```python
from build123d import *
from build123d.topology import SkipClean

# Parameters (mm, degrees)
SKETCH_1_R          = 1.55
SKETCH_1_R_2        = 4
EXTRUDE_1_DEPTH     = 3
EXTRUDE_START       = -3
SKETCH_2_R          = 2.1
EXTRUDE_3_DEPTH     = 3
FILLET_1_R          = 4
FILLET_2_R          = 314
FILLET_3_R          = 314
FILLET_4_R          = 4
CUT_EXTRUDE_2_DEPTH = 3
EXTRUDE_4_DEPTH     = 3
EXTRUDE_5_DEPTH     = 3
SKETCH_6_R          = 1.55
CUT_EXTRUDE_3_DEPTH = 10


with BuildPart() as part:
    # 草图1 → 凸台-拉伸1 (new body)
    with BuildSketch(Plane(origin=(0, 0, 0), x_dir=(1, 0, 0), z_dir=(0, 1, 0))):
        with BuildLine():
            Line((-27.819418646, 37.14796354), (-55, 11))
            Line((-55, 11), (-55, -11))
            Line((-55, -11), (-27.819418646, -37.14796354))
            ThreePointArc((-27.819418646, -37.14796354), (-23.984664844, -39.630488814), (-19.5, -40.5))
            Line((-19.5, -40.5), (-17.421399483, -40.31860482))
            Line((-17.421399483, -40.31860482), (45.042813224, -34.867481809))
            ThreePointArc((45.042813224, -34.867481809), (58.724014778, -30.74585061), (69.617928959, -21.5))
            Line((69.617928959, -21.5), (19, -21.5))
            ThreePointArc((19, -21.5), (15.464466094, -20.035533906), (14, -16.5))
            Line((14, -16.5), (14, -12.539936204))
            ThreePointArc((14, -12.539936204), (5.5, 0), (14, 12.539936204))
            Line((14, 12.539936204), (14, 16.5))
            ThreePointArc((14, 16.5), (15.464466094, 20.035533906), (19, 21.5))
            Line((19, 21.5), (69.617928959, 21.5))
            ThreePointArc((69.617928959, 21.5), (58.724014778, 30.74585061), (45.042813224, 34.867481809))
            Line((45.042813224, 34.867481809), (-17.421399483, 40.31860482))
            Line((-17.421399483, 40.31860482), (-19.5, 40.5))
            ThreePointArc((-19.5, 40.5), (-23.984664844, 39.630488814), (-27.819418646, 37.14796354))
        make_face()
        with Locations(Location((-29, -28.5, 0), (0, 0, 270))):
            Circle(SKETCH_1_R, mode=Mode.SUBTRACT)
        with Locations(Location((-19.5, -36.5, 0), (0, 0, 270))):
            Circle(SKETCH_1_R, mode=Mode.SUBTRACT)
        with Locations(Location((-19.5, -28.5, 0), (0, 0, 270))):
            Circle(SKETCH_1_R_2, mode=Mode.SUBTRACT)
        with Locations(Location((-10, -28.5, 0), (0, 0, 270))):
            Circle(SKETCH_1_R, mode=Mode.SUBTRACT)
        with Locations(Location((-19.5, -20.5, 0), (0, 0, 270))):
            Circle(SKETCH_1_R, mode=Mode.SUBTRACT)
        with Locations(Location((-46.5, 0, 0), (0, 0, 270))):
            Circle(SKETCH_1_R, mode=Mode.SUBTRACT)
        with Locations(Location((-27.5, 0, 0), (0, 0, 270))):
            Circle(SKETCH_1_R, mode=Mode.SUBTRACT)
        with Locations(Location((0, 0, 0), (0, 0, 270))):
            Circle(SKETCH_1_R, mode=Mode.SUBTRACT)
        with Locations(Location((-29, 28.5, 0), (0, 0, 270))):
            Circle(SKETCH_1_R, mode=Mode.SUBTRACT)
        with Locations(Location((-19.5, 20.5, 0), (0, 0, 270))):
            Circle(SKETCH_1_R, mode=Mode.SUBTRACT)
        with Locations(Location((-19.5, 28.5, 0), (0, 0, 270))):
            Circle(SKETCH_1_R_2, mode=Mode.SUBTRACT)
        with Locations(Location((-10, 28.5, 0), (0, 0, 270))):
            Circle(SKETCH_1_R, mode=Mode.SUBTRACT)
        with Locations(Location((-19.5, 36.5, 0), (0, 0, 270))):
            Circle(SKETCH_1_R, mode=Mode.SUBTRACT)
    extrude(amount=EXTRUDE_1_DEPTH)

    # 草图2 → 凸台-拉伸3 (add)
    with BuildSketch(Plane(origin=(0, 3, 0), x_dir=(1, 0, 0), z_dir=(0, 1, 0)).offset(EXTRUDE_START)):
        with BuildLine():
            Line((-7, 60), (-28.363974347, 36.588878709))
            ThreePointArc((-28.363974347, 36.588878709), (-26.665503977, 38.125775437), (-24.705947863, 39.311942788))
            Line((-24.705947863, 39.311942788), (-19.656872495, 39.177623495))
            Line((-19.656872495, 39.177623495), (-17.421399483, 40.31860482))
            Line((-17.421399483, 40.31860482), (17, 37.314720281))
            Line((17, 37.314720281), (17, 50))
            Line((17, 50), (17, 60))
            Line((17, 60), (-7, 60))
        make_face()
        with Locations(Location((13, 55, 0), (0, 0, 270))):
            Circle(SKETCH_2_R, mode=Mode.SUBTRACT)
        with Locations(Location((-3, 55, 0), (0, 0, 270))):
            Circle(SKETCH_2_R, mode=Mode.SUBTRACT)
    extrude_3 = extrude(amount=EXTRUDE_3_DEPTH)

    # 圆角1
    fillet_1_edges = [part.edges().sort_by_distance(p)[0] for p in [
        (17, 1.5, -37.314720281),
    ]]
    fillet(fillet_1_edges, radius=FILLET_1_R)

    # 圆角2
    # the kernel refuses this fillet: 314 mm, written as the material it adds along each edge
    with BuildSketch(Plane(origin=(-28.100791786, 0, -36.877280051), x_dir=(0.6740732257670936, 0, -0.7386645289330906), z_dir=(0, 1, 0))) as fillet_2_piece_1:
        with BuildLine():
            CenterArc((FILLET_2_R * 0.032536346624, FILLET_2_R), FILLET_2_R, 266.272924122, 3.727075878)
            Line((-FILLET_2_R * 0.0324675326171, FILLET_2_R * 0.0021149887469), (0, 0))
            Line((0, 0), (FILLET_2_R * 0.032536346624, 0))
        make_face()
    extrude(amount=3)

    # 镜向2: 凸台-拉伸3 across plane
    add(extrude_3.mirror(Plane.XY))

    # 圆角3
    # the kernel refuses this fillet: 314 mm, written as the material it adds along each edge
    with BuildSketch(Plane(origin=(-28.100791786, 0, 36.877280051), x_dir=(-0.7206636283184775, 0, -0.6932848871992288), z_dir=(0, 1, 0))) as fillet_3_piece_1:
        with BuildLine():
            CenterArc((FILLET_3_R * 0.0325363466241, FILLET_3_R), FILLET_3_R, 266.272924122, 3.727075878)
            Line((-FILLET_3_R * 0.0324675326171, FILLET_3_R * 0.0021149887469), (0, 0))
            Line((0, 0), (FILLET_3_R * 0.032536346624, 0))
        make_face()
    extrude(amount=3)

    # 圆角4
    fillet_4_edges = [part.edges().sort_by_distance(p)[0] for p in [
        (17, 1.5, 37.314720281),
    ]]
    fillet(fillet_4_edges, radius=FILLET_4_R)

    # 草图3 → 切除-拉伸2 (cut)
    with BuildSketch(Plane.XZ):
        with BuildLine():
            ThreePointArc((-8.686732059, 48.231275591), (-35.637539634, 44.178960889), (-38.911435654, 17.122558906))
            ThreePointArc((-38.911435654, 17.122558906), (-32.411561674, 15.426493388), (-30.715496156, 21.926367368))
            ThreePointArc((-30.715496156, 21.926367368), (-28.823911789, 37.55895518), (-13.252334078, 39.900292563))
            ThreePointArc((-13.252334078, 39.900292563), (-6.804041555, 41.782983067), (-8.686732059, 48.231275591))
        make_face()
    cut_extrude_2 = extrude(amount=-CUT_EXTRUDE_2_DEPTH, mode=Mode.SUBTRACT)

    # 草图4 → 凸台-拉伸4 (add)
    with SkipClean():  # the faces are left unmerged after this step: merging them gives an invalid solid
        with BuildSketch(Plane.XZ):
            with BuildLine():
                Line((-43.624805935, 21.943038922), (-41.535713139, 23.952764967))
                ThreePointArc((-41.535713139, 23.952764967), (-35.617955509, 44.199092655), (-15.534428758, 50.647781937))
                Line((-15.534428758, 50.647781937), (-13.580394358, 52.78905657))
                ThreePointArc((-13.580394358, 52.78905657), (-37.408839455, 45.943436284), (-43.624805935, 21.943038922))
            make_face()
            with BuildLine():
                ThreePointArc((-25.118289886, 40.223259732), (-28.812596517, 37.570586867), (-31.367097826, 33.807729194))
                ThreePointArc((-31.367097826, 33.807729194), (-28.219819959, 36.993214998), (-25.118289886, 40.223259732))
            make_face()
        extrude_4 = extrude(amount=-EXTRUDE_4_DEPTH)

    # 镜向9: 切除-拉伸2, 凸台-拉伸4 across plane
    with SkipClean():  # the faces are left unmerged after this step: merging them gives an invalid solid
        add(cut_extrude_2.mirror(Plane.XY), mode=Mode.SUBTRACT)
        add(extrude_4.mirror(Plane.XY))

    # 草图5 → 凸台-拉伸5 (add)
    with SkipClean():  # the faces are left unmerged after this step: merging them gives an invalid solid
        with BuildSketch(Plane(origin=(0, 3, 0), x_dir=(1, 0, 0), z_dir=(0, 1, 0)).offset(EXTRUDE_START)):
            with BuildLine():
                Line((17, 60), (61.975554983, 28.739819121))
                ThreePointArc((61.975554983, 28.739819121), (53.910011807, 32.911268872), (45.042813224, 34.867481809))
                Line((45.042813224, 34.867481809), (20.652249917, 36.995995963))
                ThreePointArc((20.652249917, 36.995995963), (18.051186651, 38.278167206), (17, 40.980851027))
                Line((17, 40.980851027), (17, 60))
            make_face()
            with BuildLine():
                Line((17, -40.980851027), (17, -60))
                Line((17, -60), (61.975554983, -28.739819121))
                ThreePointArc((61.975554983, -28.739819121), (53.910011807, -32.911268872), (45.042813224, -34.867481809))
                Line((45.042813224, -34.867481809), (20.652249917, -36.995995963))
                ThreePointArc((20.652249917, -36.995995963), (18.051186651, -38.278167206), (17, -40.980851027))
            make_face()
        extrude(amount=EXTRUDE_5_DEPTH)

    # 草图6 → 切除-拉伸3 (cut)
    with SkipClean():  # the faces are left unmerged after this step: merging them gives an invalid solid
        with BuildSketch(Plane.XZ):
            with Locations(Location((42, 31, 0), (0, 0, 270))):
                Circle(SKETCH_6_R)
            with Locations(Location((57.97553464, 25.73983326, 0), (0, 0, 270))):
                Circle(SKETCH_6_R)
        cut_extrude_3 = extrude(amount=-CUT_EXTRUDE_3_DEPTH, mode=Mode.SUBTRACT)

    # 镜向10: 切除-拉伸3 across plane
    with SkipClean():  # the faces are left unmerged after this step: merging them gives an invalid solid
        add(cut_extrude_3.mirror(Plane.XY), mode=Mode.SUBTRACT)


solid = part.part
```
Can you work these out from the model? Positions are in its coordinate system, mm. A direction names the side the tool comes from. Coordinates: 2 decimals unless noted, no trailing zeros. Loops run counter-clockwise (first coordinate to the right, second up) from the corner with the lowest first, then second, coordinate; pieces in that order, holes last.
1) I need wall thicknesses on probe 1 along X at (y, z) = (1, -36.5); probe 2 along X at (y, z) = (2.2, 28.5); probe 3 along X at (y, z) = (2.1, 31). Which ranges of each line are inside material? Lowest first, please.
2) Which directions (+Z, -Z, +X, -X, +Y, -Y) give clear straight access to the entire face, cutting with the end or side of a thin tool? Please do faces 1 (the cylindrical face through (15.43, 1.48, -20)), 2 (the cylindrical face through (13.631, 1.479, -52.997)).
3) Imagine slicing it at A-A on z = 0. List the corners of the cut face in (x, y) for me.
4) Imagine slicing it at D-D on y = 2.35. State how many separate pieces and enclosed holes the cut face has, plus the area to 3 significant figures.
5) Imagine slicing it at B-B on x = 27. List the corners of the cut face in (y, z) for me, plus the area to 3 significant figures.
6) Thinking about a two-plate mould opening in Z: for faces 3 (the cylindrical face through (-6.855, 1.479, -41.692)), 4 (the cylindrical face through (66.12, 1.48, -25.36)), 5 (the flat face through (-55, 1, 0)), which applies, pulls with the +Z half, pulls with the -Z half, needs draft (parallel to the pull), parting line crosses it, or undercut?
7) Imagine slicing it at C-C on z = -36.5. List the corners of the cut face in (x, y) for me.
8) For pin 1 (0.9 mm diameter, centred on x = 45.5, y = 1, fed in from -Z); pin 2 (1 mm diameter, centred on y = 1, z = 14, fed in from +X), each with a flat end and sliding along its axis, tell me the tip position at first contact or that it passes through.
Completed:
1. probe 1: x = -43.19 to -40.53, -29.75 to -21.05, -17.95 to 50.81
1. probe 2: x = -44.5 to -42, -32.5 to -30.55, -27.45 to -23.5, -15.5 to -11.55, -8.45 to 62.32
1. probe 3: x = -44.37 to -41.86, -32.26 to -22.62, -16.38 to 40.45, 43.55 to 58.72
2. face 1: +X, +Y, -Y
2. face 2: +Y, -Y
3. outline: (-55, 0) - (-48.05, 0) - (-48.05, 3) - (-55, 3) - close; (-44.95, 0) - (-29.05, 0) - (-29.05, 3) - (-44.95, 3) - close; (-25.95, 0) - (-1.55, 0) - (-1.55, 3) - (-25.95, 3) - close; (1.55, 0) - (5.5, 0) - (5.5, 3) - (1.55, 3) - close
4. separate pieces: 1
4. enclosed holes: 23
4. area: 7,550 mm2
5. outline: (0, -53.05) - (3, -53.05) - (3, -21.5) - (0, -21.5) - close; (0, 21.5) - (3, 21.5) - (3, 53.05) - (0, 53.05) - close
5. area: 189 mm2
6. face 3: undercut
6. face 4: pulls with the -Z half
6. face 5: needs draft
7. outline: (-43.19, 0) - (-40.53, 0) - (-40.53, 3) - (-43.19, 3) - close; (-29.75, 0) - (-21.05, 0) - (-21.05, 3) - (-29.75, 3) - close; (-17.95, 0) - (50.81, 0) - (50.81, 3) - (-17.95, 3) - close
8. pin 1: stops at z = -40.5
8. pin 2: stops at x = 14
